Autodesk Inventor part; units mm, degrees
ref_plane "YZ Plane" through (0, 0, 0) normal (1, 0, 0) x (0, 1, 0)
ref_plane "XZ Plane" through (0, 0, 0) normal (0, 1, 0) x (-1, 0, 0)
ref_plane "XY Plane" through (0, 0, 0) normal (0, 0, 1) x (1, 0, 0)
sketch "Base" plane through (0, 0, 0) normal (0, 0, 1) x (1, 0, 0)
  circle A0 centre (6.3437, -0.0043) radius 44.7044
  line L0 (-53.391, 43.8831) -> (3.4518, 87.3031)
  line L1 (3.4518, 87.3031) -> (126.7242, 46.1195)
  line L2 (21.9665, -51.542) -> (-11.8651, -109.4379)
  line L3 (134.9457, -71.4872) -> (143.2137, -54.1334)
  line L4 (44.7126, -49.2622) -> (124.7112, -76.8356)
  line L5 (44.7126, -49.2622) -> (21.9665, -51.542)
  line L6 (126.7242, 46.1195) -> (143.2137, -54.1334)
  line L7 (134.9457, -71.4872) -> (124.7112, -76.8356)
  line L8 (-30.3614, -103.0627) -> (-11.8651, -109.4379)
  line L9 (-30.3614, -103.0627) -> (-19.8027, -31.8971)
  line L10 (-54.6035, 18.8674) -> (-53.391, 43.8831)
  line L11 (-54.6035, 18.8674) -> (-19.8027, -31.8971)
  line L12 (-94.1669, 0) -> (182.7771, 0) construction
  circle A1 centre (6.3437, -0.0043) radius 3
  circle A2 centre (103.8642, -35.9814) radius 3
  line L13 (126.7242, 46.1195) -> (-19.8027, -31.8971) construction
  line L14 (3.4518, 87.3031) -> (33.3396, -50.4021) construction
  line L15 (-53.9972, 31.3753) -> (126.7242, 46.1195) construction
  line L16 (134.969, -4.007) -> (-37.2031, -6.5149) construction
  line L17 (-21.1132, -106.2503) -> (39.5241, 75.2519) construction
  line L18 (78.4642, -60.8955) -> (78.4642, 62.2425) construction
  line L19 (21.9665, -51.542) -> (126.7242, 46.1195) construction
  line L20 (0, 0) -> (-53.391, 43.8831) construction
  circle A3 centre (-20.3518, 21.9373) radius 3
  circle A4 centre (6.3437, -0.0043) radius 34.5555 construction
  circle A5 centre (-26.006, -12.1525) radius 3
  circle A6 centre (0.6895, -34.0941) radius 3
  circle A7 centre (33.0392, -21.9459) radius 3
  circle A8 centre (38.6934, 12.1439) radius 3
  circle A9 centre (11.9979, 34.0855) radius 3
  line L21 (113.2722, 38.9571) -> (102.0622, 32.9885) construction
  line L22 (111.8623, 41.6052) -> (100.6522, 35.6365)
  line L23 (103.4721, 30.3404) -> (114.6821, 36.3091)
  arc A10 (114.6821, 36.3091) -> (111.8623, 41.6052) centre (113.2722, 38.9571) ccw
  arc A11 (100.6522, 35.6365) -> (103.4721, 30.3404) centre (102.0622, 32.9885) ccw
  line L24 (119.5611, -4.2314) -> (106.8611, -4.2314) construction
  line L25 (119.5611, -1.2314) -> (106.8611, -1.2314)
  line L26 (106.8611, -7.2314) -> (119.5611, -7.2314)
  arc A12 (119.5611, -7.2314) -> (119.5611, -1.2314) centre (119.5611, -4.2314) ccw
  arc A13 (106.8611, -1.2314) -> (106.8611, -7.2314) centre (106.8611, -4.2314) ccw
  line L27 (6.6843, 72.4098) -> (9.378, 59.9988) construction
  line L28 (3.7525, 71.7735) -> (6.4462, 59.3625)
  line L29 (12.3097, 60.6351) -> (9.616, 73.0462)
  arc A14 (9.616, 73.0462) -> (3.7525, 71.7735) centre (6.6843, 72.4098) ccw
  arc A15 (6.4462, 59.3625) -> (12.3097, 60.6351) centre (9.378, 59.9988) ccw
  line L30 (-16.2839, -91.795) -> (-12.2597, -79.7494) construction
  line L31 (-13.4385, -92.7456) -> (-9.4142, -80.7)
  line L32 (-15.1051, -78.7988) -> (-19.1293, -90.8444)
  arc A16 (-19.1293, -90.8444) -> (-13.4385, -92.7456) centre (-16.2839, -91.795) ccw
  arc A17 (-9.4142, -80.7) -> (-15.1051, -78.7988) centre (-12.2597, -79.7494) ccw
  line L33 (78.4642, -44.7756) -> (78.4642, -32.0756) construction
  line L34 (75.4642, -44.7756) -> (75.4642, -32.0756)
  line L35 (81.4642, -32.0756) -> (81.4642, -44.7756)
  arc A18 (75.4642, -44.7756) -> (81.4642, -44.7756) centre (78.4642, -44.7756) ccw
  arc A19 (81.4642, -32.0756) -> (75.4642, -32.0756) centre (78.4642, -32.0756) ccw
  line L36 (-38.6678, 39.9478) -> (-26.0099, 40.9805) construction
  line L37 (-38.4239, 36.9578) -> (-25.766, 37.9905)
  line L38 (-26.2538, 43.9706) -> (-38.9118, 42.9379)
  arc A20 (-38.9118, 42.9379) -> (-38.4239, 36.9578) centre (-38.6678, 39.9478) ccw
  arc A21 (-25.766, 37.9905) -> (-26.2538, 43.9706) centre (-26.0099, 40.9805) ccw
  line L39 (45.5702, -29.5373) -> (54.8596, -20.8771) construction
  line L40 (47.6159, -31.7316) -> (56.9053, -23.0715)
  line L41 (52.8139, -18.6828) -> (43.5245, -27.3429)
  arc A22 (43.5245, -27.3429) -> (47.6159, -31.7316) centre (45.5702, -29.5373) ccw
  arc A23 (56.9053, -23.0715) -> (52.8139, -18.6828) centre (54.8596, -20.8771) ccw
  line L42 (-38.6678, 39.9478) -> (-53.391, 43.8831) construction
  circle A24 centre (122.4612, -51.192) radius 3
  point P0 (107.6672, 35.9728)
  point P1 (113.2111, -4.2314)
  point P2 (8.0311, 66.2043)
  point P3 (-14.2718, -85.7722)
  point P4 (78.4642, -38.4256)
  point P5 (-32.3389, 40.4642)
  point P6 (50.2149, -25.2072)
  dimension "d48" = 69.111
  dimension "d1" = 89.4088
  dimension "d2" = 55.568
  dimension "d3" = 37.094
  dimension "d4" = 120.3
  dimension "d5" = 81.561
  dimension "d6" = 160.982
  dimension "d7" = 133.392
  dimension "d8" = 143.066
  dimension "d9" = 145.185
  dimension "d10" = 124.151
  dimension "d11" = 130.15
  dimension "d12" = 142.793
  dimension "d13" = 117.814
  dimension "d14" = 19.5642
  dimension "d15" = 25.0158
  dimension "d16" = 71.529
  dimension "d17" = 61.5478
  dimension "d18" = 129.9699
  dimension "d19" = 101.6
  dimension "d20" = 19.2227
  dimension "d21" = 11.5477
  dimension "d22" = 84.6172
  dimension "d23" = 67.056
  dimension "d24" = 22.86
  dimension "d25" = 39.5986
  dimension "d26" = 71.1371
  dimension "d29" = 6
  dimension "d30" = 6
  dimension "d31" = 48.26
  dimension "d32" = 6
  dimension "d35" = 360
  dimension "d37" = 6
  dimension "d38" = 6
  dimension "d39" = 15.24
  dimension "d40" = 12.7
  dimension "d41" = 15.24
  dimension "d43" = 15.24
  dimension "d44" = 15.24
  dimension "d45" = 15.24
  dimension "d46" = 15.7016
  dimension "d49" = 140.583
  dimension "d50" = 4.2314
  dimension "d51" = 91.5631
  dimension "d52" = 12.1439
  dimension "d53" = 0
  dimension "d60" = 126.024
  dimension "d61" = 155.259
  dimension "d63" = 15.24
  dimension "d64" = 12.0647
  dimension "d67" = 25.4
  dimension "d68" = 31.75
  dimension "d69" = 6
  dimension "d70" = 20
  dimension "d71" = 20
  dimension "d72" = 3
  dimension "d73" = 3
  dimension "d74" = 3
  dimension "d75" = 3
  dimension "d76" = 3
  dimension "d77" = 3
  dimension "d78" = 3
  dimension "d79" = 3
  dimension "d80" = 3
  dimension "d81" = 3
extrude "Plate1" add sketch "Base" along normal blind 5 contours A0 L9 L11 | A0 L11 L10 L0 L1 L6 L3 L7 L4 L5 L2 L8 L9 | A5 picked at (-13.3863, 3.3874)
fillet "OutsideFilletsFeature" radius 6.35 12 edges at (126.7242, 46.1195, 2.5) (3.4518, 87.3031, 2.5) (143.2137, -54.1334, 2.5) (134.9457, -71.4872, 2.5) (124.7112, -76.8356, 2.5) (-11.8651, -109.4379, 2.5) (44.7126, -49.2622, 2.5) (21.9665, -51.542, 2.5) (-30.3614, -103.0627, 2.5) (-19.8027, -31.8971, 2.5) (-54.6035, 18.8674, 2.5) (-53.391, 43.8831, 2.5)
sketch "HandleAttachment" plane through (0, 0, 0) normal (0, 0, -1) x (-1, 0, 0)
  circle A0 centre (-122.4612, -51.192) radius 3
  point P0 (0, 0)
equation "\"d41\" = d39"
equation "\"d43\" = d39"
equation "\"d44\" = d43"
equation "\"d45\" = d43"
equation "\"d47\" = Thickness"
properties part number "UpperLeg2"
The model under review builds one solid part; all positions refer to its coordinate system, in mm. A direction names the side the tool comes from. Give positions to 0.01 mm unless a question says otherwise; leave off trailing zeros. Write each loop counter-clockwise with the first axis right and the second up, starting at its lowest first coordinate (ties: lowest second). Pieces come first, ordered by that corner, then holes. Notation, with made-up numbers: M 34.25,24.25 L 74.25,24.25 A20 cw 74.25,58.25 Z; hole C 0,54 d8. An arc over 180 degrees is marked long. Write item = value, one per line. Start each with the question number.
Q1. Clearance check with flat-ended pins moving along their axes: pin 1 (2 mm diameter, centred on x = 113, z = 1.5, fed in from -Y); pin 2 (7 mm diameter, centred on x = 0.69, y = -34.09, fed in from -Z); pin 3 (2 mm diameter, centred on x = 71, z = 3.5, fed in from +Y); pin 4 (3 mm diameter, centred on x = 39.5, z = 3.5, fed in from +Y). State where each tip first meets the part, or that it passes through.
Q2. For line 1 (X direction, y = -34.5, z = 3.9); line 2 (X direction, y = -29.5, z = 1.85); line 3 (X direction, y = 40, z = 3.85), list the stretches that pass through material, from the lowest coordinate up.
Q3. We need section C-C (y = 6). State the section outline as (x, z) points, plus the area to 3 significant figures.
Q4. Machinability: for faces 5 (the face through (-24.944, -66.549, 2.465)), 6 (the face through (-32.49, 43.46, 2.46)), 7 (the face through (-54.024, 30.829, 2.465)), which of the approach directions +Z, -Z, +X, -X, +Y, -Y give a long, thin tool a straight path to every point of the face, cutting with its end or side? Answer none if there is none.
Q5. We need section B-B (x = 85.5). State the section outline as (y, z) points, plus the area to 3 significant figures.
Q6. We need section A-A (z = 3.75). Give the number of separate pieces and of enclosed holes in the cut face, plus the area to 3 significant figures.
Q7. Mouldability with a two-part tool opening along X and no side actions: class faces 1 (the face through (125.944, 45.392, 2.535)), 2 (the face through (-21.14, -106.24, 2.46)), 3 (the face through (100.867, -36.113, 2.465)), 4 (the face through (5.08, 65.65, 2.46)) as released by +X, released by -X, zero draft, split by the parting line, or undercut.
Result set:
q1.pin_1 = -73.14
q1.pin_2 = 0
q1.pin_3 = 65.07
q1.pin_4 = 75.76
q2.line_1 = -20.19 to -2.28, 3.66 to 75.46, 81.46 to 101.26, 106.47 to 139.98
q2.line_2 = -21.45 to 42.57, 50.01 to 76.93, 80 to 139.16
q2.line_3 = -53.58 to -41.67, -23.17 to 108.85, 116.09 to 127.73
q3.outline = M -45.78,0 L 133.32,0 L 133.32,5 L -45.78,5 Z
q3.area = 896 mm2
q4.face_5 = +Z, -Z, -X
q4.face_6 = +Z, -Z
q4.face_7 = +Z, -Z, -X, +Y
q5.outline = M -63.32,0 L 59.89,0 L 59.89,5 L -63.32,5 Z
q5.area = 616 mm2
q6.separate_pieces = 1
q6.enclosed_holes = 15
q6.area = 22,600 mm2
q7.face_1 = released by +X
q7.face_2 = released by -X
q7.face_3 = undercut
q7.face_4 = undercut
